```python
from build123d import *

# Parameters (mm, degrees)
F0_W     = 38.1
F0_H     = 38.1
F1_DEPTH = 25.4
F3_DEPTH = 25.4
F4_W     = 12.7
F4_H     = 6.35
F5_DEPTH = 25.4


with BuildPart() as f1:
    # F0 (on Front) → F1 (new body)
    with BuildSketch(Plane.XZ):
        with Locations((-19.05, 19.05)):
            Rectangle(F0_W, F0_H)
    extrude(amount=F1_DEPTH)

    # F2 (on face) → F3 (cut)
    with BuildSketch(Plane.XZ.offset(25.4)):
        Polygon((-38.1, 38.1), (-38.1, 0), (-23.319498, 38.1), align=None)
        Polygon((-12.6649, 38.1), (0, 0), (0, 38.1), align=None)
    extrude(amount=-F3_DEPTH, mode=Mode.SUBTRACT)

    # F4 (on face) → F5 (cut)
    with BuildSketch(Plane.XZ.offset(25.4)):
        with Locations((-17.371559, 3.175)):
            Rectangle(F4_W, F4_H)
    extrude(amount=-F5_DEPTH, mode=Mode.SUBTRACT)


solid = f1.part
```
Geometry check sheet. Reference: the model listing, model coordinates, mm. A direction names the side the tool comes from. Coordinates: 2 decimals unless noted, no trailing zeros. Order: outer loops, then holes, each group sorted by start corner. A loop starts at its lowest first (then second) coordinate and runs counter-clockwise, first axis right, second up.
Q1. Sectioned sample at B-B on x = -15. Record the cut outline in (y, z), and give its area (3 significant figures).
Reply:
outline: (-25.4, 6.35) - (0, 6.35) - (0, 38.1) - (-25.4, 38.1) - close
area: 806 mm2
Q2. Tool access check on faces 1 (the face through (-17, -13, 6.35)), 2 (the face through (-18, -13, 38.1)). Record the directions out of +Z, -Z, +X, -X, +Y, -Y that give a thin tool (end or side, any length) a straight path to the whole face; none if there is none.
Reply:
face 1: -Z, +Y, -Y
face 2: +Z, +X, -X, +Y, -Y
Q3. Sectioned sample at C-C on z = 34. Record the cut outline in (x, y).
Reply:
outline: (-24.91, -25.4) - (-11.3, -25.4) - (-11.3, 0) - (-24.91, 0) - close
Q4. Draft check along X on faces 3 (the face through (-11.022, -13, 3)), 4 (the face through (-30.813, -12.878, 18.783)), 5 (the face through (-19, 0, 15)), 6 (the face through (-6.421, -12.878, 19.317)). Enter one of: released by +X, released by -X, zero draft, split by the parting line, or undercut.
Reply:
face 3: undercut
face 4: released by -X
face 5: zero draft
face 6: released by +X
Q5. Sectioned sample at A-A on y = -16. Record the cut outline in (x, z), and give its area (3 significant figures).
Reply:
outline: (-38.1, 0) - (-23.72, 0) - (-23.72, 6.35) - (-11.02, 6.35) - (-11.02, 0) - (0, 0) - (-12.66, 38.1) - (-23.32, 38.1) - close
area: 848 mm2
Q6. Thickness scan on probe 1 along X at (y, z) = (-15, 5.5); probe 2 along Z at (x, y) = (-20.5, -6.75); probe 3 along X at (y, z) = (-21, 27.5). Record the ranges inside material, lowest first.
Reply:
probe 1: x = -35.97 to -23.72, -11.02 to -1.83
probe 2: z = 6.35 to 38.1
probe 3: x = -27.43 to -9.14
Q7. Depth check by flat-ended pin: pin 1 Ø3 at (y, z) = (-13, 4.5) entering from -X; pin 2 Ø4 at (x, z) = (-24, 31) entering from +Y; pin 3 Ø1 at (y, z) = (-20.5, 9.5) entering from +X; pin 4 Ø6 at (y, z) = (-9.5, 17) entering from -X. Enter the tip coordinate at first touch or a pass-through.
Reply:
pin 1: stops at x = -36.94
pin 2: stops at y = 0
pin 3: stops at x = -2.99
pin 4: stops at x = -32.67
